For this review, take the finished solid that the model builds, in its own axes (mm). Face numbers are marked on the shaded views. Round coordinates to 2 decimals unless told otherwise and drop trailing zeros. Write each loop counter-clockwise with the first axis right and the second up, starting at its lowest first coordinate (ties: lowest second). Pieces come first, ordered by that corner, then holes. Notation, with made-up numbers: M 44,1.25 L 72,1.25 A8 ccw 72,12.25 Z; hole C 2.5,-25.75 d3. An arc over 180 degrees is marked long. Write each question's results on one line, items separated by ' | '. Start each with the question number.
```python
from build123d import *

# Parameters (mm, degrees)
SKETCH1_W           = 47.55
SKETCH1_H           = 47.55
SKETCH1_R           = 1.7
SKETCH1_R_2         = 16
BOSS_EXTRUDE1_DEPTH = 12
SKETCH2_R           = 16
SKETCH2_R_2         = 11
BOSS_EXTRUDE2_DEPTH = 2
FILLET1_R           = 5


with BuildPart() as part:
    # Sketch1 → Boss-Extrude1 (new body)
    with BuildSketch(Plane(origin=(0, 0, 0), x_dir=(1, 0, 0), z_dir=(0, 1, 0))):
        Rectangle(SKETCH1_W, SKETCH1_H)
        with Locations(Location((-15.5, 15.5, 0), (0, 0, 270))):
            Circle(SKETCH1_R, mode=Mode.SUBTRACT)
        with Locations(Location((15.5, 15.5, 0), (0, 0, 270))):
            Circle(SKETCH1_R, mode=Mode.SUBTRACT)
        with Locations(Location((15.5, -15.5, 0), (0, 0, 270))):
            Circle(SKETCH1_R, mode=Mode.SUBTRACT)
        with Locations(Location((-15.5, -15.5, 0), (0, 0, 270))):
            Circle(SKETCH1_R, mode=Mode.SUBTRACT)
        with Locations(Location((0, 0, 0), (0, 0, 270))):
            Circle(SKETCH1_R_2, mode=Mode.SUBTRACT)
    extrude(amount=BOSS_EXTRUDE1_DEPTH)

    # Sketch2 → Boss-Extrude2 (add)
    with BuildSketch(Plane.XZ):
        with Locations(Location((0, 0, 0), (0, 0, 270))):
            Circle(SKETCH2_R)
        with Locations(Location((0, 0, 0), (0, 0, 270))):
            Circle(SKETCH2_R_2, mode=Mode.SUBTRACT)
    extrude(amount=-BOSS_EXTRUDE2_DEPTH)

    # Fillet1
    fillet1_edges = [part.edges().sort_by_distance(p)[0] for p in [
        (23.775, 6, 23.775),
        (-23.775, 6, 23.775),
        (-23.775, 6, -23.775),
        (23.775, 6, -23.775),
    ]]
    fillet(fillet1_edges, radius=FILLET1_R)


solid = part.part
```
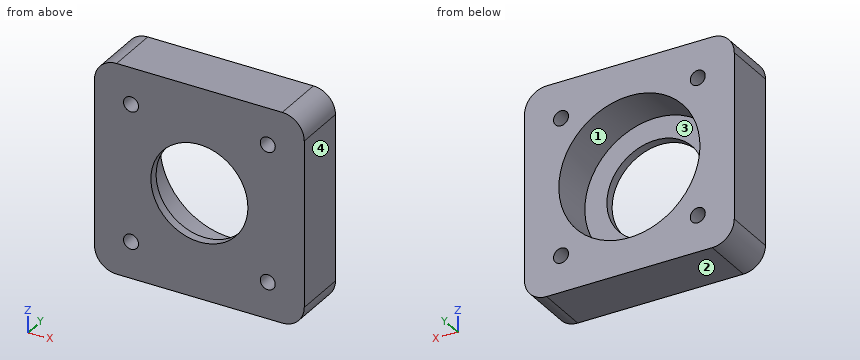
Item 1: Insertion check: P1, Ø3, axis at x = -15.5, z = 15.5, coming from the -Y side. The pin has a flat end and moves straight along its axis. Give the tip position at first contact, or say it passes through.
Item 2: We need section C-C on z = -2.5. State the section outline as (x, y) points (3 decimals).
Item 3: We need section B-B on x = 2. State the section outline as (y, z) points (1 decimal), then the cut area to 3 significant figures.
Item 4: Mouldability with a two-part tool opening along X and no side actions: class the marked faces 1, 2, 3 and 4 as pulls with the +X half, pulls with the -X half, needs draft (parallel to the pull), parting line crosses it, or undercut.
Item 5: We need section A-A on y = 3.25. State the section outline as (x, z) points (3 decimals).
Item 6: We need section D-D on x = 12. State the section outline as (y, z) points (3 decimals), then the cut area to 3 significant figures.
Item 7: For probe 1 along Z at (x, y) = (14.5, 9) (3 decimals); probe 2 along X at (y, z) = (1.5, 0) (3 decimals); probe 3 along X at (y, z) = (3.75, -14) (3 decimals), list the stretches that pass through material, from the lowest coordinate up.
Numbers:
1) P1: passes through
2) outline: M -23.775,0 L -10.712,0 L -10.712,2 L -15.803,2 L -15.803,12 L -23.775,12 Z; M 10.712,0 L 23.775,0 L 23.775,12 L 15.803,12 L 15.803,2 L 10.712,2 Z
3) outline: M 0,-23.8 L 12,-23.8 L 12,-15.9 L 2,-15.9 L 2,-10.8 L 0,-10.8 Z; M 0,10.8 L 2,10.8 L 2,15.9 L 12,15.9 L 12,23.8 L 0,23.8 Z | area: 210 mm^2
4) face 1: undercut | face 2: needs draft | face 3: undercut | face 4: pulls with the +X half
5) outline: M -23.775,-18.775 A5 ccw -18.775,-23.775 L 18.775,-23.775 A5 ccw 23.775,-18.775 L 23.775,18.775 A5 ccw 18.775,23.775 L -18.775,23.775 A5 ccw -23.775,18.775 Z; hole C -15.5,-15.5 d3.4; hole C -15.5,15.5 d3.4; hole C 0,0 d32; hole C 15.5,-15.5 d3.4; hole C 15.5,15.5 d3.4
6) outline: M 0,-23.775 L 12,-23.775 L 12,-10.583 L 2,-10.583 L 2,10.583 L 12,10.583 L 12,23.775 L 0,23.775 Z | area: 359 mm^2
7) probe 1: z = -23.775 to -16.875, -14.125 to -6.764, 6.764 to 14.125, 16.875 to 23.775 | probe 2: x = -23.775 to -11, 11 to 23.775 | probe 3: x = -23.775 to -16.3, -14.7 to -7.746, 7.746 to 14.7, 16.3 to 23.775
